The model under review builds one solid part; all positions refer to its coordinate system, in mm. A direction names the side the tool comes from. Coordinates: 2 decimals unless noted, no trailing zeros. Loops run counter-clockwise (first coordinate to the right, second up) from the corner with the lowest first, then second, coordinate; pieces in that order, holes last. Notation, with made-up numbers: M 30,-30 L 44,-30 A10 ccw 44,-20 Z; hole C 20.25,83.25 d5. An arc over 180 degrees is marked long. Use CSV: the item, a comma, the result in double quotes. Start each with the question number.
from build123d import *

# Parameters (mm, degrees)
SKETCH1_W           = 101.6
SKETCH1_H           = 34.925
BOSS_EXTRUDE2_DEPTH = 26.9875
BOSS_EXTRUDE3_DEPTH = 17.4625


with BuildPart() as part:
    # Sketch1 → Boss-Extrude2 (new body)
    with BuildSketch(Plane.XY):
        Polygon((12.7, 19.910607408), (50.8, 0), (-50.8, 0), align=None)
        with Locations((0, -17.4625)):
            Rectangle(SKETCH1_W, SKETCH1_H)
    extrude(amount=BOSS_EXTRUDE2_DEPTH)

    # Sketch3 → Boss-Extrude3 (add)
    with BuildSketch(Plane.XY.offset(26.9875)):
        Polygon((-50.8, 0), (0, -11.346798656), (0, -34.925), (-50.8, -34.925), align=None)
    extrude(amount=BOSS_EXTRUDE3_DEPTH)


solid = part.part
1. For faces 1 (the flat face through (-50.8, -18, 22)), 2 (the flat face through (12, -7, 26.988)), 3 (the flat face through (0, -23, 36)), list the 3-axis set-ups (+Z, -Z, +X, -X, +Y, -Y) from which the entire face can be reached by the end or side of a thin tool; tool diameter is ignored.
2. Add section B-B (z = 9). Write out the cut boundary in (x, y) (3 decimals), plus the area to 3 significant figures.
3. Add section A-A (y = -21.5). Write out the cut boundary in (x, z), plus the area to 3 significant figures.
4. To check wall thickness, follow line 1 along Z through (x, y) = (10.5, -20); line 2 along X through (y, z) = (-20.5, 42.5); line 3 along Y through (x, z) = (20, 11.5) (3 decimals). State the ranges of each line that lie inside material, in increasing order.
5. Add section D-D (z = 31). Write out the cut boundary in (x, y) (3 decimals), plus the area to 3 significant figures.
6. Insertion check: pin 1 Ø3 at (y, z) = (13, 8.5) entering from +X; pin 2 Ø8.5 at (y, z) = (-22, 32.5) entering from +X; pin 3 Ø2 at (x, z) = (20.5, 24) entering from +Y. Each pin has a flat end and moves straight along its axis. Give the tip position at first contact, or say it passes through.
Solved:
1,face 1,"+Z, -Z, -X, +Y, -Y"
1,face 2,"+Z, +X, +Y"
1,face 3,"+Z, +X, +Y, -Y"
2,outline,"M -50.8,-34.925 L 50.8,-34.925 L 50.8,0 L 12.7,19.911 L -50.8,0 Z"
2,area,"4,560 mm^2"
3,outline,"M -50.8,0 L 50.8,0 L 50.8,26.99 L 0,26.99 L 0,44.45 L -50.8,44.45 Z"
3,area,"3,630 mm^2"
4,line 1,"z = 0 to 26.99"
4,line 2,"x = -50.8 to 0"
4,line 3,"y = -34.925 to 16.096"
5,outline,"M -50.8,-34.925 L 0,-34.925 L 0,-11.347 L -50.8,0 Z"
5,area,"1,490 mm^2"
6,pin 1,"stops at x = 28.79"
6,pin 2,"stops at x = 0"
6,pin 3,"stops at y = 16.36"
